Geometry check sheet. Reference: the model listing, model coordinates, mm. Face numbers are marked on the shaded views. A direction names the side the tool comes from. Coordinates: 2 decimals unless noted, no trailing zeros. Loops run counter-clockwise (first coordinate to the right, second up) from the corner with the lowest first, then second, coordinate; pieces in that order, holes last.
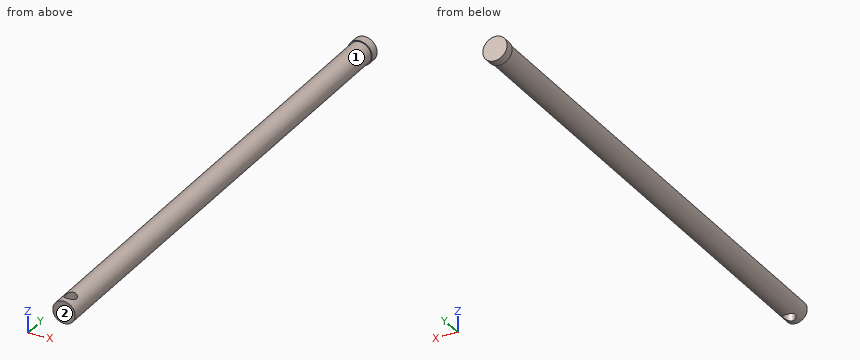
from build123d import *

# Parameters (mm, degrees)
SKETCH1_R                  = 4.953
BOSS_EXTRUDE1_DEPTH        = 228.6
BOSS_EXTRUDE2_START        = -3.81
SKETCH2_R                  = 5.3975
SKETCH2_R_2                = 4.953
BOSS_EXTRUDE2_DEPTH        = 3.81
F_6_0_204_DIAMETER_HOLE1_D = 5.1816


with BuildPart() as part:
    # Sketch1 → Boss-Extrude1 (new body)
    with BuildSketch(Plane(origin=(0, 0, 0), x_dir=(1, 0, 0), z_dir=(0, 1, 0))):
        with Locations(Location((0, 0, 0), (0, 0, 270))):
            Circle(SKETCH1_R)
    extrude(amount=BOSS_EXTRUDE1_DEPTH)

    # Sketch2 → Boss-Extrude2 (add)
    with BuildSketch(Plane(origin=(0, 228.6, 0), x_dir=(1, 0, 0), z_dir=(0, 1, 0)).offset(BOSS_EXTRUDE2_START)):
        with Locations(Location((0, 0, 0), (0, 0, 270))):
            Circle(SKETCH2_R)
        with Locations(Location((0, 0, 0), (0, 0, 270))):
            Circle(SKETCH2_R_2, mode=Mode.SUBTRACT)
    extrude(amount=BOSS_EXTRUDE2_DEPTH)

    # #6 (0.204) Diameter Hole1 (through all)
    with Locations(Plane.XY.offset(4.953)):
        with Locations((0, 5.08)):
            Hole(F_6_0_204_DIAMETER_HOLE1_D / 2)


solid = part.part
1) Depth check by flat-ended pin: pin 1 (6 mm diameter, centred on y = 123, z = 0, fed in from +X); pin 2 (2 mm diameter, centred on x = -2, y = 94.5, fed in from -Z); pin 3 (6 mm diameter, centred on x = 3, y = 202, fed in from +Z). Enter the tip coordinate at first touch or a pass-through.
Data:
pin 1: stops at x = 4.95
pin 2: stops at z = -4.85
pin 3: stops at z = 4.95
2) Section check B-B on z = 0. Record the cut outline in (x, y).
Data:
outline: (-5.4, 224.79) - (-4.95, 224.79) - (-4.95, 0) - (4.95, 0) - (4.95, 224.79) - (5.4, 224.79) - (5.4, 228.6) - (-5.4, 228.6) - close; hole circle Ø5.18 at (0, 5.08)
3) Section check C-C on y = 187. Record the cut outline in (x, z).
Data:
outline: circle Ø9.91 at (0, 0)
4) Section check A-A on x = 0. Record the cut outline in (y, z).
Data:
outline: (0, -4.95) - (2.49, -4.95) - (2.49, 4.95) - (0, 4.95) - close; (7.67, -4.95) - (224.79, -4.95) - (224.79, -5.4) - (228.6, -5.4) - (228.6, 5.4) - (224.79, 5.4) - (224.79, 4.95) - (7.67, 4.95) - close
5) Material ranges on probe 1 along Y at (x, z) = (0, 1.25); probe 2 along X at (y, z) = (5.08, 0.5); probe 3 along Y at (x, z) = (4.75, -2.25), recorded low to high.
Data:
probe 1: y = 0 to 2.49, 7.67 to 228.6
probe 2: x = -4.93 to -2.59, 2.59 to 4.93
probe 3: y = 224.79 to 228.6
6) Section check D-D on y = 5.08. Record the cut outline in (x, z).
Data:
outline: (-2.59, -4.22) - (-2.59, 4.22) arc R4.95 ccw to start; (2.59, -4.22) arc R4.95 ccw to (2.59, 4.22) - close
7) Access from +Z, -Z, +X, -X, +Y, -Y to the whole of each face (thin tool, end or side, straight path). Record for the marked faces 1 and 2.
Data:
face 1: -Y
face 2: +Z, -Z, +X, -X, -Y
